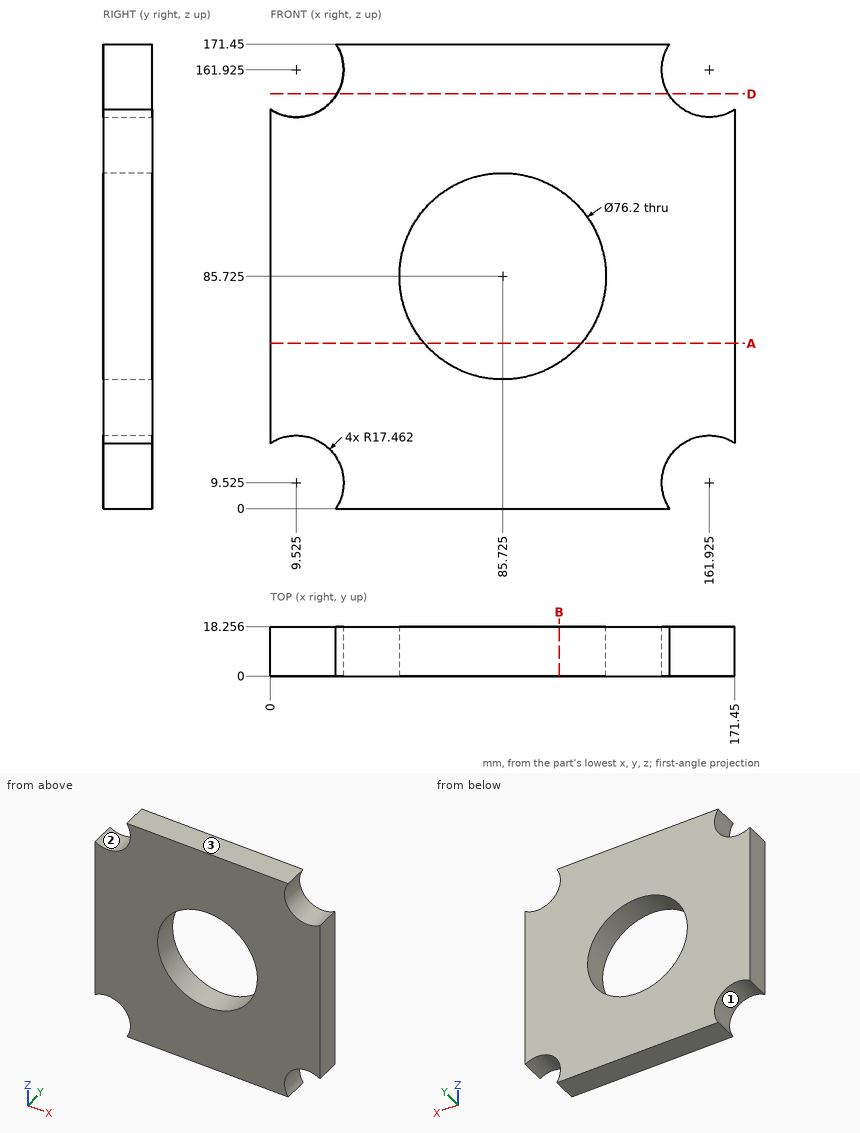
Study the drawing (mm; zero at the part's minimum x, y, z) and answer. Coordinates: 2 decimals unless noted, no trailing zeros. Write each loop counter-clockwise with the first axis right and the second up, starting at its lowest first coordinate (ties: lowest second). Pieces come first, ordered by that corner, then holes. Notation, with made-up numbers: M 50,-27 L 97,-27 A19 cw 97,-3 Z; hole C 34,-14 d8. An arc over 180 degrees is marked long. Use one line per item in the form item = value.
Item 1: Find section A-A, the plane z = 61. Give the vertices of the cut face in (x, y), plus the area to 3 significant figures.
Model answer:
outline = M 0,0 L 56.74,0 L 56.74,18.26 L 0,18.26 Z; M 114.71,0 L 171.45,0 L 171.45,18.26 L 114.71,18.26 Z
area = 2,070 mm2
Item 2: The mould has two halves that part along X. Classify the marked faces 1, 2 and 3: released by +X, released by -X, zero draft, split by the parting line, or undercut.
Model answer:
face_1 = undercut
face_2 = undercut
face_3 = zero draft
Item 3: Find section B-B, the plane x = 106.5. Give the vertices of the cut face in (y, z).
Model answer:
outline = M 0,0 L 18.26,0 L 18.26,53.79 L 0,53.79 Z; M 0,117.66 L 18.26,117.66 L 18.26,171.45 L 0,171.45 Z
Item 4: Find the intervals of material crossed by probe 1 along Z at (x, y) = (162.5, 6.25); probe 2 along X at (y, z) = (7.25, 62.5); probe 3 along X at (y, z) = (7.5, 83.5), in increasing order.
Model answer:
probe_1 = 26.98 to 144.47
probe_2 = 0 to 55.52, 115.93 to 171.45
probe_3 = 0 to 47.69, 123.76 to 171.45
Item 5: Find section D-D, the plane z = 153. Give the vertices of the cut face in (x, y) (1 decimal).
Model answer:
outline = M 24.5,0 L 146.9,0 L 146.9,18.3 L 24.5,18.3 Z
